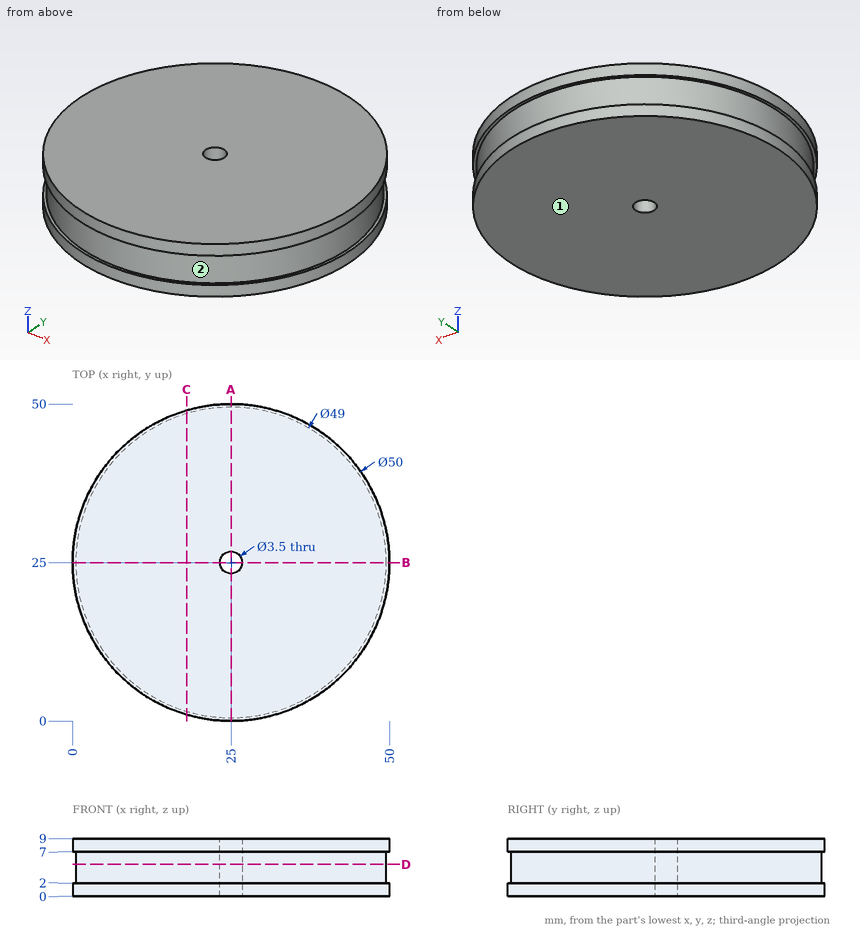
Study the drawing (mm; zero at the part's minimum x, y, z) and answer. Coordinates: 2 decimals unless noted, no trailing zeros. Loops run counter-clockwise (first coordinate to the right, second up) from the corner with the lowest first, then second, coordinate; pieces in that order, holes last. Notation, with made-up numbers: (-30, -12) -> (-1, -12) arc R31 cw to (-1, 21) -> close; hole circle Ø7 at (-20, 27). An arc over 180 degrees is marked (long way). Answer in a Markdown table with one row per item. Add a question column.
1. Flat-ended cylindrical pins translate along their axes: P1, Ø3, axis at x = 5.5, z = 6.5, coming from the -Y side; P2, Ø1.5, axis at x = 39.5, z = 4, coming from the +Y side. Find the tip coordinate at first contact, or state that the pin passes through.
2. Consider line 1 (Y direction, x = 25, z = 1.25); line 2 (Y direction, x = 26, z = 6); line 3 (Y direction, x = 20, z = 7.75). Determine where each line is inside the solid, lowest interval first. Write a range as [from, to].
3. The part is cut by section A-A, the plane x = 25. Write down the section's boundary in (y, z).
4. Determine the mould class of the marked faces 1 and 2 for opening direction X: +X half, -X half, draft (parallel to the pull), parting line (faces both ways), or undercut.
5. The part is cut by section D-D, the plane z = 5. Write down the section's boundary in (x, y), then the cut area to 3 significant figures.
6. The part is cut by section C-C, the plane x = 18. Write down the section's boundary in (y, z).
Answer below:
| question | item | result |
|---|---|---|
| 1 | P1 | y = 7.74 |
| 1 | P2 | y = 45.28 |
| 2 | line 1 | [0, 23.25], [26.75, 50] |
| 2 | line 2 | [0.52, 23.56], [26.44, 49.48] |
| 2 | line 3 | [0.51, 49.49] |
| 3 | outline | (0, 0) -> (23.25, 0) -> (23.25, 9) -> (0, 9) -> (0, 7) -> (0.5, 7) -> (0.5, 2) -> (0, 2) -> close; (26.75, 0) -> (50, 0) -> (50, 2) -> (49.5, 2) -> (49.5, 7) -> (50, 7) -> (50, 9) -> (26.75, 9) -> close |
| 4 | face 1 | draft |
| 4 | face 2 | parting line |
| 5 | outline | circle Ø49 at (25, 25); hole circle Ø3.5 at (25, 25) |
| 5 | area | 1,880 mm2 |
| 6 | outline | (1, 0) -> (49, 0) -> (49, 2) -> (48.48, 2) -> (48.48, 7) -> (49, 7) -> (49, 9) -> (1, 9) -> (1, 7) -> (1.52, 7) -> (1.52, 2) -> (1, 2) -> close |
